For this review, take the finished solid that the model builds, in its own axes (mm). A direction names the side the tool comes from. Coordinates: 2 decimals unless noted, no trailing zeros. Write each loop counter-clockwise with the first axis right and the second up, starting at its lowest first coordinate (ties: lowest second). Pieces come first, ordered by that corner, then holes. Notation, with made-up numbers: (-8.5, 44) -> (50.5, 44) arc R12 ccw to (50.5, 49) -> close; hole circle Ø11 at (-35, 67). An arc over 180 degrees is marked (long way). One line per item, written item: value. Start each with the question number.
1) For pin 1 Ø12 at (x, y) = (14.5, 29.5) entering from +Z; pin 2 Ø4.5 at (x, z) = (15, 10) entering from -Y, all flat-tipped, find the tip position at first contact; note any pin that passes through.
2) Add section A-A (z = 9.25). State the section outline as (x, y) points, and give its area (3 significant figures).
3) Machinability: for faces 4 (the cylindrical face through (8.44, 40.5, 10.94)), 5 (the flat face through (0, -10, 7)), 6 (the flat face through (10, 14, 0)), which of the approach directions +Z, -Z, +X, -X, +Y, -Y give a long, thin tool a straight path to every point of the face, cutting with its end or side? Answer none if there is none.
4) Add section D-D (z = 3.25). State the section outline as (x, y) points.
5) For probe 1 along Y at (x, z) = (10, 11); probe 2 along X at (y, z) = (-15, 11.5); probe 3 along Y at (x, z) = (10, 3), list the stretches that pass through material, from the lowest coordinate up. Write a range as from..to.
6) Add section C-C (x = 10). State the section outline as (y, z) points, and give its area (3 significant figures).
7) Add section B-B (y = 28.6). State the section outline as (x, z) points, and give its area (3 significant figures).
8) Mouldability with a two-part tool opening along X and no side actions: class faces 1 (the flat face through (-8, 12, 7)), 2 (the cylindrical face through (11.172, 37.523, 3.451)), 3 (the flat face through (10, 14, 15)) as released by +X, released by -X, zero draft, split by the parting line, or undercut.
from build123d import *

# Parameters (mm, degrees)
CROQUIS1_R              = 12
SALIENTE_EXTRUIR1_DEPTH = 15
CROQUIS3_R              = 12
CROQUIS3_R_2            = 9
SALIENTE_EXTRUIR2_DEPTH = 7


with BuildPart() as part:
    # Croquis1 → Saliente-Extruir1 (new body)
    with BuildSketch(Plane.XY):
        with BuildLine():
            Line((0, -20), (0, 0))
            Line((0, 0), (20, 0))
            Line((20, 0), (20, -20))
            Line((20, -20), (28, -20))
            Line((28, -20), (28, 43))
            ThreePointArc((28, 43), (26.535533906, 46.535533906), (23, 48))
            Line((23, 48), (-3, 48))
            ThreePointArc((-3, 48), (-6.535533906, 46.535533906), (-8, 43))
            Line((-8, 43), (-8, -20))
            Line((-8, -20), (0, -20))
        make_face()
        with Locations((10, 28.6)):
            Circle(CROQUIS1_R, mode=Mode.SUBTRACT)
    extrude(amount=SALIENTE_EXTRUIR1_DEPTH)

    # Croquis3 → Saliente-Extruir2 (add)
    with BuildSketch(Plane(origin=(0, 0, 0), x_dir=(-1, 0, 0), z_dir=(0, 0, -1))):
        with Locations((-10, 28.6)):
            Circle(CROQUIS3_R)
        with Locations((-10, 28.6)):
            Circle(CROQUIS3_R_2, mode=Mode.SUBTRACT)
    extrude(amount=-SALIENTE_EXTRUIR2_DEPTH)


solid = part.part
Numbers:
1. pin 1: z = 7
1. pin 2: y = 0
2. outline: (-8, -20) -> (0, -20) -> (0, 0) -> (20, 0) -> (20, -20) -> (28, -20) -> (28, 43) arc R5 ccw to (23, 48) -> (-3, 48) arc R5 ccw to (-8, 43) -> close; hole circle Ø24 at (10, 28.6)
2. area: 1,580 mm²
3. face 4: +Z
3. face 5: +Z, -Z, -Y
3. face 6: -Z, +X, -X, +Y, -Y
4. outline: (-8, -20) -> (0, -20) -> (0, 0) -> (20, 0) -> (20, -20) -> (28, -20) -> (28, 43) arc R5 ccw to (23, 48) -> (-3, 48) arc R5 ccw to (-8, 43) -> close; hole circle Ø18 at (10, 28.6)
5. probe 1: 0..16.6, 40.6..48
5. probe 2: -8..0, 20..28
5. probe 3: 0..19.6, 37.6..48
6. outline: (0, 0) -> (19.6, 0) -> (19.6, 7) -> (16.6, 7) -> (16.6, 15) -> (0, 15) -> close; (37.6, 0) -> (48, 0) -> (48, 15) -> (40.6, 15) -> (40.6, 7) -> (37.6, 7) -> close
6. area: 402 mm²
7. outline: (-8, 0) -> (1, 0) -> (1, 7) -> (-2, 7) -> (-2, 15) -> (-8, 15) -> close; (19, 0) -> (28, 0) -> (28, 15) -> (22, 15) -> (22, 7) -> (19, 7) -> close
7. area: 222 mm²
8. face 1: released by -X
8. face 2: undercut
8. face 3: zero draft
